Geometry: final body of the model. Coordinates: model frame, mm. Face numbers are marked on the shaded views. A direction names the side the tool comes from. Give positions to 0.01 mm unless a question says otherwise; leave off trailing zeros. Loops run counter-clockwise (first coordinate to the right, second up) from the corner with the lowest first, then second, coordinate; pieces in that order, holes last. Notation, with made-up numbers: (80, -28.75) -> (110, -28.75) arc R19 ccw to (110, -9.75) -> close; hole circle Ø2 at (-9, 68.25). An arc over 180 degrees is marked (long way). Answer in a Markdown table with one row per item. Add a question column.
1) Line query: line 1 (Z direction, x = -17, y = 0.5); line 2 (Y direction, x = 16.5, z = 6.5); line 3 (X direction, y = -9, z = 15.5). Output: solid intervals per line, ascending. Write a range as from..to.
2) Section query D-D (z = 17). Return the cut outline in (x, y), plus the area to 3 significant figures.
3) First-contact query: P1, Ø1.5, axis at x = -17.5, z = 8.5, coming from the +Y side; P2, Ø1.5, axis at x = 1.5, z = 17.5, coming from the -Y side; P3, Ø2, axis at x = 12, y = 5.5, coming from the +Z side. Flat tips, straight axial feed; report the tip coordinate or a pass-through.
4) Section query A-A (x = 0). Return the cut outline in (y, z), plus the area to 4 significant figures.
5) Access query for the marked faces 1, 2 and 3. Directions: +Z, -Z, +X, -X, +Y, -Y. A direction counts if a zero-diameter tool reaches every point of the face in a straight line with its end or side. Return the directions, or none.
6) Section query C-C (y = 10). Return the cut outline in (x, z), plus the area to 3 significant figures.
7) Section query B-B (z = 2.5). Return the cut outline in (x, y).
```python
from build123d import *

# Parameters (mm, degrees)
SKETCH1_W           = 45
SKETCH1_H           = 30
BOSS_EXTRUDE1_DEPTH = 16
SKETCH2_W           = 7
SKETCH2_H           = 3.5
BOSS_EXTRUDE2_DEPTH = 5
FILLET1_R           = 10


with BuildPart() as part:
    # Sketch1 → Boss-Extrude1 (new body)
    with BuildSketch(Plane.XY):
        Rectangle(SKETCH1_W, SKETCH1_H)
    extrude(amount=BOSS_EXTRUDE1_DEPTH)

    # Sketch2 → Boss-Extrude2 (add)
    with BuildSketch(Plane.XY.offset(16)):
        Rectangle(SKETCH2_W, SKETCH2_H)
    extrude(amount=BOSS_EXTRUDE2_DEPTH)

    # Fillet1
    fillet1_edges = [part.edges().sort_by_distance(p)[0] for p in [
        (22.5, -15, 8),
        (-22.5, -15, 8),
        (-22.5, 15, 8),
        (22.5, 15, 8),
    ]]
    fillet(fillet1_edges, radius=FILLET1_R)


solid = part.part
```
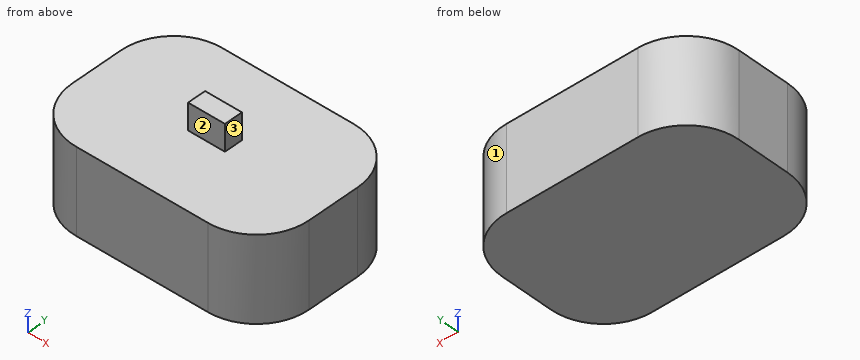
Evaluation:
| question | item | result |
|---|---|---|
| 1 | line 1 | 0..16 |
| 1 | line 2 | -14.17..14.17 |
| 1 | line 3 | -21.67..21.67 |
| 2 | outline | (-3.5, -1.75) -> (3.5, -1.75) -> (3.5, 1.75) -> (-3.5, 1.75) -> close |
| 2 | area | 24.5 mm² |
| 3 | P1 | y = 14.05 |
| 3 | P2 | y = -1.75 |
| 3 | P3 | z = 16 |
| 4 | outline | (-15, 0) -> (15, 0) -> (15, 16) -> (1.75, 16) -> (1.75, 21) -> (-1.75, 21) -> (-1.75, 16) -> (-15, 16) -> close |
| 4 | area | 497.5 mm² |
| 5 | face 1 | +Z, -Z, +X, +Y |
| 5 | face 2 | +Z, +X, -X, -Y |
| 5 | face 3 | +Z, +X, +Y, -Y |
| 6 | outline | (-21.16, 0) -> (21.16, 0) -> (21.16, 16) -> (-21.16, 16) -> close |
| 6 | area | 677 mm² |
| 7 | outline | (-22.5, -5) arc R10 ccw to (-12.5, -15) -> (12.5, -15) arc R10 ccw to (22.5, -5) -> (22.5, 5) arc R10 ccw to (12.5, 15) -> (-12.5, 15) arc R10 ccw to (-22.5, 5) -> close |
